from build123d import *

# Parameters (mm, degrees)
BOSS_EXTRUDE1_DEPTH = 6
CUT_EXTRUDE1_START  = -2
CUT_EXTRUDE1_DEPTH  = 4
SKETCH2_7_R         = 1.150000003
CUT_EXTRUDE3_DEPTH  = 10


with BuildPart() as part:
    # Sketch1 → Boss-Extrude1 (new body)
    with BuildSketch(Plane.XY):
        with BuildLine():
            Line((-31.185934329, 10), (-26.901486948, 10))
            ThreePointArc((-26.901486948, 10), (0, 28.7), (26.901486948, 10))
            Line((26.901486948, 10), (31.185934329, 10))
            ThreePointArc((31.185934329, 10), (0, 32.75), (-31.185934329, 10))
        make_face()
        with BuildLine():
            ThreePointArc((-26.901486948, -10), (-28.7, 0), (-26.901486948, 10))
            Line((-26.901486948, 10), (-31.185934329, 10))
            ThreePointArc((-31.185934329, 10), (-32.75, 0), (-31.185934329, -10))
            Line((-31.185934329, -10), (-26.901486948, -10))
        make_face()
        with BuildLine():
            ThreePointArc((26.901486948, -10), (0, -28.7), (-26.901486948, -10))
            Line((-26.901486948, -10), (-31.185934329, -10))
            ThreePointArc((-31.185934329, -10), (0, -32.75), (31.185934329, -10))
            Line((31.185934329, -10), (26.901486948, -10))
        make_face()
        with BuildLine():
            Line((31.185934329, 10), (26.901486948, 10))
            ThreePointArc((26.901486948, 10), (28.246793406, 5.080222662), (28.7, 0))
            ThreePointArc((28.7, 0), (28.246793406, -5.080222662), (26.901486948, -10))
            Line((26.901486948, -10), (31.185934329, -10))
            ThreePointArc((31.185934329, -10), (32.356621033, -5.060788017), (32.75, 0))
            ThreePointArc((32.75, 0), (32.356621033, 5.060788017), (31.185934329, 10))
        make_face()
    extrude(amount=BOSS_EXTRUDE1_DEPTH)

    # Sketch2 → Cut-Extrude1 (cut)
    with BuildSketch(Plane.XY.offset(6).offset(CUT_EXTRUDE1_START)):
        with BuildLine():
            ThreePointArc((-20.861737651, 25.245799694), (-23.157747084, 23.157747084), (-25.245799694, 20.861737651))
            Line((-25.245799694, 20.861737651), (-23.40529254, 19.021230496))
            ThreePointArc((-23.40529254, 19.021230496), (-22.821141725, 18.562842449), (-22.144742459, 18.256516136))
            ThreePointArc((-22.144742459, 18.256516136), (-20.29396462, 20.29396462), (-18.256516136, 22.144742459))
            ThreePointArc((-18.256516136, 22.144742459), (-18.562842449, 22.821141725), (-19.021230496, 23.40529254))
            Line((-19.021230496, 23.40529254), (-20.861737651, 25.245799694))
        make_face()
        with BuildLine():
            Line((20.861737651, 25.245799694), (19.021230496, 23.40529254))
            ThreePointArc((19.0212305, 23.405292536), (18.562842453, 22.821141721), (18.25651614, 22.144742456))
            ThreePointArc((18.25651614, 22.144742456), (20.29396462, 20.29396462), (22.144742456, 18.25651614))
            ThreePointArc((22.144742456, 18.25651614), (22.821141721, 18.562842453), (23.405292536, 19.0212305))
            Line((23.40529254, 19.021230496), (25.245799694, 20.861737651))
            ThreePointArc((25.245799694, 20.861737651), (23.157747084, 23.157747084), (20.861737651, 25.245799694))
        make_face()
        with BuildLine():
            Line((-23.40529254, -19.021230496), (-25.245799694, -20.861737651))
            ThreePointArc((-25.245799694, -20.861737651), (-23.157747084, -23.157747084), (-20.861737651, -25.245799694))
            Line((-20.861737651, -25.245799694), (-19.021230496, -23.40529254))
            ThreePointArc((-19.021230492, -23.405292544), (-18.562842445, -22.821141728), (-18.256516131, -22.144742463))
            ThreePointArc((-18.256516131, -22.144742463), (-20.29396462, -20.29396462), (-22.144742463, -18.256516131))
            ThreePointArc((-22.144742463, -18.256516131), (-22.821141728, -18.562842445), (-23.405292544, -19.021230492))
        make_face()
        with BuildLine():
            Line((25.245799694, -20.861737651), (23.40529254, -19.021230496))
            ThreePointArc((23.40529254, -19.021230496), (22.821141725, -18.562842449), (22.144742459, -18.256516136))
            ThreePointArc((22.144742459, -18.256516136), (20.29396462, -20.29396462), (18.256516136, -22.144742459))
            ThreePointArc((18.256516136, -22.144742459), (18.562842449, -22.821141725), (19.021230496, -23.40529254))
            Line((19.021230496, -23.40529254), (20.861737651, -25.245799694))
            ThreePointArc((20.861737651, -25.245799694), (23.157747084, -23.157747084), (25.245799694, -20.861737651))
        make_face()
    extrude(amount=CUT_EXTRUDE1_DEPTH, mode=Mode.SUBTRACT)

    # Sketch2_7 → Cut-Extrude3 (cut)
    with BuildSketch(Plane.XY.offset(6)):
        with Locations((-21.213261518, -21.213261518)):
            Circle(SKETCH2_7_R)
        with Locations((-21.213261518, 21.213261518)):
            Circle(SKETCH2_7_R)
        with Locations((21.213261518, 21.213261518)):
            Circle(SKETCH2_7_R)
        with Locations((21.213261518, -21.213261518)):
            Circle(SKETCH2_7_R)
    extrude(amount=-CUT_EXTRUDE3_DEPTH, mode=Mode.SUBTRACT)


solid = part.part
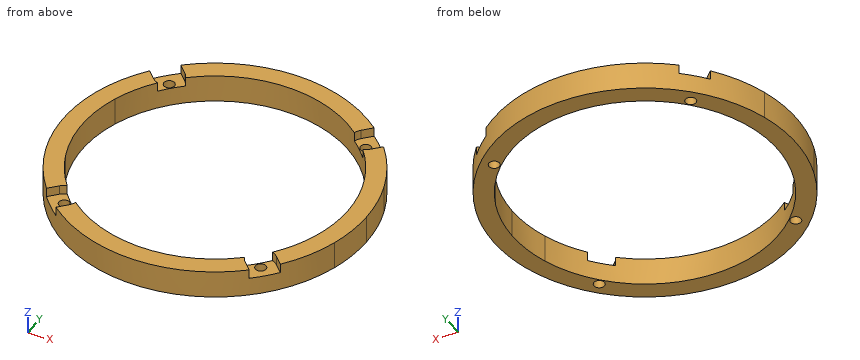
Source: CAD feature listing. Evaluate the final solid. Frame: model axes, mm. Give positions to 0.01 mm unless a question says otherwise; leave off trailing zeros. Write each loop counter-clockwise with the first axis right and the second up, starting at its lowest first coordinate (ties: lowest second). Pieces come first, ordered by that corner, then holes. Notation, with made-up numbers: (63.5, 86.5) -> (112.5, 86.5) arc R21 cw to (112.5, 112.5) -> close; hole circle Ø6 at (-11, 85). An arc over 180 degrees is marked (long way). Return JSON: item names as keys, results as strings. Group by question number.
1. Section D-D, the plane z = 1.6. Output: boundary loops of the cut face in (x, y), then the cut area to 3 significant figures.
2. Section C-C, the plane x = 2.5. Output: boundary loops of the cut face in (y, z).
3. Pin query (flat end, axial travel): pin 1 Ø3.5 at (x, y) = (-21, -20.5) entering from +Z; pin 2 Ø1.5 at (x, z) = (-26, 3) entering from -Y; pin 3 Ø1.5 at (y, z) = (-23, 2.5) entering from -X. Return the tip coordinate at first contact, or that it passes through.
4. Material intervals for line 1 (Y direction, x = -21.5, z = 2.55); line 2 (Y direction, x = -21, z = 3.6); line 3 (X direction, y = -17, z = 1.3), sorted ascending. Write a range as from..to.
5. Section A-A, the plane z = 5.2. Output: boundary loops of the cut face in (x, y).
6. Section B-B, the plane y = -17. Output: boundary loops of the cut face in (x, z).
Determined:
{
 "1": {"outline": "circle Ø65.5 at (0, 0); hole circle Ø57.4 at (0, 0); hole circle Ø2.3 at (-21.21, -21.21); hole circle Ø2.3 at (-21.21, 21.21); hole circle Ø2.3 at (21.21, -21.21); hole circle Ø2.3 at (21.21, 21.21)", "area": "765 mm2"},
 "2": {"outline": "(-32.65, 0) -> (-28.59, 0) -> (-28.59, 6) -> (-32.65, 6) -> close; (28.59, 0) -> (32.65, 0) -> (32.65, 6) -> (28.59, 6) -> close"},
 "3": {"pin 1": "stops at z = 4", "pin 2": "stops at y = -20.86", "pin 3": "stops at x = -24.03"},
 "4": {"line 1": "y = -24.7..-22.33, -20.1..-19.01, 19.01..20.1, 22.33..24.7", "line 2": "y = -25.13..-22.34, -20.08..-19.56, 19.56..20.08, 22.34..25.13", "line 3": "x = -27.99..-23.12, 23.12..27.99"},
 "5": {"outline": "(-25.25, -20.86) -> (-23.41, -19.02) arc R3.1 cw to (-22.14, -18.26) arc R28.7 cw to (-22.14, 18.26) arc R3.1 cw to (-23.41, 19.02) -> (-25.25, 20.86) arc R32.75 ccw to start; (-20.86, -25.25) arc R32.75 ccw to (20.86, -25.25) -> (19.02, -23.41) arc R3.1 cw to (18.26, -22.14) arc R28.7 cw to (-18.26, -22.14) arc R3.1 cw to (-19.02, -23.41) -> close; (-20.86, 25.25) -> (-19.02, 23.41) arc R3.1 cw to (-18.26, 22.14) arc R28.7 cw to (18.26, 22.14) arc R3.1 cw to (19.02, 23.41) -> (20.86, 25.25) arc R32.75 ccw to start; (22.14, -18.26) arc R3.1 cw to (23.41, -19.02) -> (25.25, -20.86) arc R32.75 ccw to (25.25, 20.86) -> (23.41, 19.02) arc R3.1 cw to (22.14, 18.26) arc R28.7 cw to start"},
 "6": {"outline": "(-27.99, 0) -> (-23.12, 0) -> (-23.12, 6) -> (-27.99, 6) -> close; (23.12, 0) -> (27.99, 0) -> (27.99, 6) -> (23.12, 6) -> close"}
}
